```python
from build123d import *

# Parameters (mm, degrees)
SKETCH1_R           = 10
BOSS_EXTRUDE1_DEPTH = 15
BOSS_EXTRUDE2_DEPTH = 25
SKETCH3_W           = 40
SKETCH3_H           = 10
CUT_EXTRUDE1_DEPTH  = 71.710678119


with BuildPart() as part:
    # Sketch1 → Boss-Extrude1 (new body)
    with BuildSketch(Plane(origin=(0, 0, 0), x_dir=(-1, 0, 0), z_dir=(0, 1, 0))):
        Polygon((-30, -50), (30, -50), (30, 25), (-15, 25), (-30, 10), align=None)
        with Locations(Location((0, 0, 0), (0, 0, 90))):
            Circle(SKETCH1_R, mode=Mode.SUBTRACT)
    extrude(amount=BOSS_EXTRUDE1_DEPTH)

    # Sketch2 → Boss-Extrude2 (add)
    with BuildSketch(Plane(origin=(0, 15, 0), x_dir=(-1, 0, 0), z_dir=(0, 1, 0))):
        Polygon((-30, -50), (-30, -30), (30, -30), (30, -50), (20, -50), (20, -40), (-20, -40), (-20, -50), align=None)
    extrude(amount=BOSS_EXTRUDE2_DEPTH)

    # Sketch3 → Cut-Extrude1 (cut, through all)
    with BuildSketch(Plane(origin=(0, 40, 0), x_dir=(-1, 0, 0), z_dir=(0, 1, 0))):
        with Locations((0, -45)):
            Rectangle(SKETCH3_W, SKETCH3_H)
    extrude(amount=-CUT_EXTRUDE1_DEPTH, mode=Mode.SUBTRACT)


solid = part.part
```
The model under review builds one solid part; all positions refer to its coordinate system, in mm. A direction names the side the tool comes from. Round coordinates to 2 decimals unless told otherwise and drop trailing zeros. Loops run counter-clockwise (first coordinate to the right, second up) from the corner with the lowest first, then second, coordinate; pieces in that order, holes last. Notation, with made-up numbers: (57.5, 24) -> (79.5, 24) arc R8 ccw to (79.5, 30) -> close; hole circle Ø10 at (-12.5, 19.25). An arc over 180 degrees is marked (long way). Answer as a JSON object with one key per item and string values. Group by question number.
1) For faces 1 (the face through (-6.2, 15, -8.2)), 2 (the face through (-25, 20, -50)), 3 (the face through (20, 20, -45)), list the 3-axis set-ups (+Z, -Z, +X, -X, +Y, -Y) from which the entire face can be reached by the end or side of a thin tool; tool diameter is ignored.
2) We need section A-A on x = 0. Write out the cut boundary in (y, z), then the cut area to 3 significant figures.
3) Mouldability with a two-part tool opening along X and no side actions: class faces 4 (the face through (0, 0, -12)), 5 (the face through (0, 20, -40)), 6 (the face through (30, 11, -27)), 7 (the face through (-30, 11, -20)) as released by +X, released by -X, zero draft, split by the parting line, or undercut.
4) We need section D-D on z = -42.5. Write out the cut boundary in (x, y).
5) For line 1 (X direction, y = 9.5, z = -45.5); line 2 (X direction, y = 11.75, z = 0); line 3 (Z direction, x = 5.5, y = 23.5), list the stretches that pass through material, from the lowest coordinate up. Write a range as [from, to].
6) We need section C-C on y = 9.5. Write out the cut boundary in (x, z).
7) We need section B-B on z = -6. Write out the cut boundary in (x, y).
8) For pin 1 Ø12 at (y, z) = (26, 4.5) entering from -X; pin 2 Ø3 at (x, z) = (-1, -41) entering from -Y; pin 3 Ø16.5 at (x, z) = (-2, -0.5) entering from +Y; pin 4 Ø8 at (x, y) = (-22.5, 29) entering from +Z, all flat-tipped, find the tip position at first contact; note any pin that passes through.
Result set:
{
 "1": {"face 1": "+Z, +X, -X, +Y", "face 2": "-Z, +X, -X, +Y, -Y", "face 3": "-Z, +Y, -Y"},
 "2": {"outline": "(0, -40) -> (40, -40) -> (40, -30) -> (15, -30) -> (15, -10) -> (0, -10) -> close; (0, 10) -> (15, 10) -> (15, 25) -> (0, 25) -> close", "area": "925 mm²"},
 "3": {"face 4": "zero draft", "face 5": "undercut", "face 6": "released by +X", "face 7": "released by -X"},
 "4": {"outline": "(-30, 0) -> (-20, 0) -> (-20, 40) -> (-30, 40) -> close; (20, 0) -> (30, 0) -> (30, 40) -> (20, 40) -> close"},
 "5": {"line 1": "[-30, -20], [20, 30]", "line 2": "[-30, -10], [10, 30]", "line 3": "[-40, -30]"},
 "6": {"outline": "(-30, -50) -> (-20, -50) -> (-20, -40) -> (20, -40) -> (20, -50) -> (30, -50) -> (30, 10) -> (15, 25) -> (-30, 25) -> close; hole circle Ø20 at (0, 0)"},
 "7": {"outline": "(-30, 0) -> (-8, 0) -> (-8, 15) -> (-30, 15) -> close; (8, 0) -> (30, 0) -> (30, 15) -> (8, 15) -> close"},
 "8": {"pin 1": "through", "pin 2": "y = 0", "pin 3": "y = 15", "pin 4": "z = -30"}
}
